from build123d import *

# Parameters (mm, degrees)
F0_W     = 279.4
F0_H     = 304.8
F1_DEPTH = 25.4
F2_W     = 279.4
F2_H     = 25.4
F3_DEPTH = 25.4
F4_W     = 279.4
F4_H     = 12.7
F5_DEPTH = 12.7
F6_W     = 6.35
F6_H     = 260.35
F7_DEPTH = 12.7
F8_W     = 12.7
F8_H     = 196.85
F9_DEPTH = 12.7


with BuildPart() as f1:
    # F0 (on Right) → F1 (new body)
    with BuildSketch(Plane.YZ):
        with Locations((-139.7, 152.4)):
            Rectangle(F0_W, F0_H)
    extrude(amount=F1_DEPTH)

    # F2 (on Right) → F3 (join)
    with BuildSketch(Plane.YZ):
        with Locations((-139.7, -12.7)):
            Rectangle(F2_W, F2_H)
    extrude(amount=F3_DEPTH)

    # F4 (on face) → F5 (cut)
    with BuildSketch(Plane(origin=(0, 0, 0), x_dir=(0, -1, 0), z_dir=(-1, 0, 0))):
        with Locations((139.7, 292.1)):
            Rectangle(F4_W, F4_H)
    extrude(amount=-F5_DEPTH, mode=Mode.SUBTRACT)

    # F6 (on face) → F7 (join)
    with BuildSketch(Plane.XZ.offset(279.4)):
        with Locations((15.875, 130.175)):
            Rectangle(F6_W, F6_H)
    extrude(amount=F7_DEPTH)

    # F8 (on face) → F9 (join)
    with BuildSketch(Plane(origin=(0, 0, 0), x_dir=(-1, 0, 0), z_dir=(0, 1, 0))):
        with Locations((-12.7, 161.925)):
            Rectangle(F8_W, F8_H)
    extrude(amount=F9_DEPTH)


solid = f1.part
The model under review builds one solid part; all positions refer to its coordinate system, in mm. A direction names the side the tool comes from. Coordinates: 2 decimals unless noted, no trailing zeros. Loops run counter-clockwise (first coordinate to the right, second up) from the corner with the lowest first, then second, coordinate; pieces in that order, holes last. Notation, with made-up numbers: (50, 77) -> (60, 77) arc R13 ccw to (60, 90) -> close; hole circle Ø10 at (3, 50.5). An arc over 180 degrees is marked (long way). Use a Markdown table: item, result. Add a question column.
1. Clearance check with flat-ended pins moving along their axes: pin 1 Ø10 at (x, z) = (4, 54) entering from -Y; pin 2 Ø4 at (y, z) = (-288.5, 69.5) entering from +X; pin 3 Ø3 at (x, y) = (16, -283.5) entering from +Z. State where each tip first meets the part, or that it passes through.
2. Machinability: for faces 1 (the face through (12.7, -286, 128)), 2 (the face through (6, -138, 298.45)), 3 (the face through (19.05, -286, 128)), 4 (the face through (13, 6, 63.5)), which of the approach directions +Z, -Z, +X, -X, +Y, -Y give a long, thin tool a straight path to every point of the face, cutting with its end or side? Answer none if there is none.
3. Add section A-A on z = 33.5. Write out the cut boundary in (x, y), plus the area to 3 significant figures.
4. Add section C-C on z = 183.5. Write out the cut boundary in (x, y), plus the area to 3 significant figures.
5. To check wall thickness, follow line 1 (Z direction, x = 3.75, y = -24.5); line 2 (Y direction, x = 10.5, z = 184); line 3 (Y direction, x = 22.75, z = 81). State the ranges of each line that lie inside material, in increasing order.
6. Draft analysis for pull direction Z (two halves, no side actions). For faces 5 (the face through (13, 6, 260.35)), 6 (the face through (6, -138, 285.75)), 7 (the face through (19.05, 6, 161)), 8 (the face through (12.7, -138, 292)), state which applies: pulls with the +Z half, pulls with the -Z half, needs draft (parallel to the pull), parting line crosses it, or undercut.
7. Add section D-D on z = 279. Write out the cut boundary in (x, y).
8. Add section B-B on y = -29.5. Write out the cut boundary in (x, z).
Returned:
| question | item | result |
|---|---|---|
| 1 | pin 1 | stops at y = -279.4 |
| 1 | pin 2 | stops at x = 19.05 |
| 1 | pin 3 | stops at z = 260.35 |
| 2 | face 1 | +Z, -Z, -X, -Y |
| 2 | face 2 | -X, +Y, -Y |
| 2 | face 3 | +Z, -Z, +X, -Y |
| 2 | face 4 | -Z, +X, -X, +Y |
| 3 | outline | (0, -279.4) -> (12.7, -279.4) -> (12.7, -292.1) -> (19.05, -292.1) -> (19.05, -279.4) -> (25.4, -279.4) -> (25.4, 0) -> (0, 0) -> close |
| 3 | area | 7,180 mm² |
| 4 | outline | (0, -279.4) -> (12.7, -279.4) -> (12.7, -292.1) -> (19.05, -292.1) -> (19.05, -279.4) -> (25.4, -279.4) -> (25.4, 0) -> (19.05, 0) -> (19.05, 12.7) -> (6.35, 12.7) -> (6.35, 0) -> (0, 0) -> close |
| 4 | area | 7,340 mm² |
| 5 | line 1 | z = -25.4 to 285.75, 298.45 to 304.8 |
| 5 | line 2 | y = -279.4 to 12.7 |
| 5 | line 3 | y = -279.4 to 0 |
| 6 | face 5 | pulls with the +Z half |
| 6 | face 6 | undercut |
| 6 | face 7 | needs draft |
| 6 | face 8 | undercut |
| 7 | outline | (0, -279.4) -> (25.4, -279.4) -> (25.4, 0) -> (0, 0) -> close |
| 8 | outline | (0, -25.4) -> (25.4, -25.4) -> (25.4, 304.8) -> (0, 304.8) -> (0, 298.45) -> (12.7, 298.45) -> (12.7, 285.75) -> (0, 285.75) -> close |
